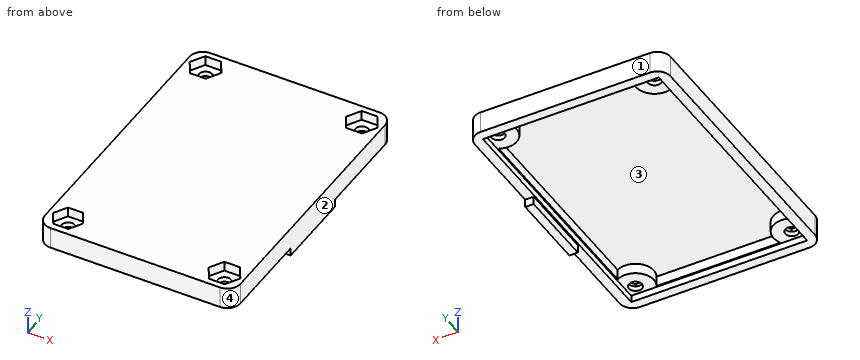
Autodesk Inventor part; units mm, degrees
ref_plane "YZ Plane" through (0, 0, 0) normal (1, 0, 0) x (0, 1, 0)
ref_plane "XZ Plane" through (0, 0, 0) normal (0, 1, 0) x (-1, 0, 0)
ref_plane "XY Plane" through (0, 0, 0) normal (0, 0, 1) x (1, 0, 0)
ref_plane "РабПлоскость1" through (0, 0, 0) normal (0, 0, 1) x (1, 0, 0)
sketch "Эскиз1" plane through (0, 0, 0) normal (0, 0, 1) x (1, 0, 0)
  line L0 (22.5, 29.5) -> (22.5, 9)
  arc A0 (22.5, 29.5) -> (19.5, 32.5) centre (19.5, 29.5) ccw
  line L1 (-19.5, 32.5) -> (19.5, 32.5)
  arc A1 (-19.5, 32.5) -> (-22.5, 29.5) centre (-19.5, 29.5) ccw
  line L2 (-22.5, -29.5) -> (-22.5, 29.5)
  arc A2 (-22.5, -29.5) -> (-19.5, -32.5) centre (-19.5, -29.5) ccw
  line L3 (19.5, -32.5) -> (-19.5, -32.5)
  arc A3 (19.5, -32.5) -> (22.5, -29.5) centre (19.5, -29.5) ccw
  line L4 (22.5, -9) -> (22.5, -29.5)
  line L5 (20, -9) -> (22.5, -9)
  line L6 (20, -25) -> (20, -9)
  line L7 (18, -25) -> (20, -25)
  arc A4 (18, -25) -> (15, -28) centre (18, -28) ccw
  line L8 (15, -30) -> (15, -28)
  line L9 (-15, -30) -> (15, -30)
  line L10 (-15, -28) -> (-15, -30)
  arc A5 (-15, -28) -> (-18, -25) centre (-18, -28) ccw
  line L11 (-20, -25) -> (-18, -25)
  line L12 (-20, 25) -> (-20, -25)
  line L13 (-18, 25) -> (-20, 25)
  arc A6 (-18, 25) -> (-15, 28) centre (-18, 28) ccw
  line L14 (-15, 30) -> (-15, 28)
  line L15 (15, 30) -> (-15, 30)
  line L16 (15, 28) -> (15, 30)
  arc A7 (15, 28) -> (18, 25) centre (18, 28) ccw
  line L17 (20, 25) -> (18, 25)
  line L18 (20, 9) -> (20, 25)
  line L19 (22.5, 9) -> (20, 9)
  circle A8 centre (-18, -28) radius 1.5
  circle A9 centre (-18, 28) radius 1.5
  circle A10 centre (18, 28) radius 1.5
  circle A11 centre (18, -28) radius 1.5
  line L20 (22.5, 9) -> (22.5, -9)
  line L21 (20, 9) -> (20, -9.6142)
  circle A12 centre (18, 28) radius 4.2426
  circle A13 centre (18, -28) radius 4.2426
  circle A14 centre (-18, -28) radius 4.2426
  circle A15 centre (-18, 28) radius 4.2426
  point P0 (0, 0)
  point P1 (-14.2583, -30)
  point P2 (-20, -24.2583)
  point P3 (-20, 24.2583)
  point P4 (-14.2583, 30)
  point P5 (20, -24.2583)
  point P6 (14.2583, -30)
  point P7 (14.2583, 30)
  point P8 (20, 24.2583)
extrude "Выдавливание1" add sketch "Эскиз1" along normal blind 4 contours L0 L19 L18 A12 L15 A15 L12 A14 L9 A13 L6 L5 L4 A3 L3 A2 L2 A1 L1 A0 | L20 L5 L21 L19 | A12 L15 L16 A7 L17 L18 | L18 L17 A7 L16 L15 A12 | A15 L12 L13 A6 L14 L15 | L15 L14 A6 L13 L12 A15 | A13 L9 L8 A4 L7 L6 | L6 L7 A4 L8 L9 A13 | A14 L9 L10 A5 L11 L12 | L12 L11 A5 L10 L9 A14
sketch "Эскиз2" plane through (0, 0, 4) normal (0, 0, 1) x (1, 0, 0)
  circle A0 centre (18, 28) radius 1.5
  circle A1 centre (18, -28) radius 1.5
  circle A2 centre (-18, 28) radius 1.5
  line L0 (16.1813, 24.85) -> (14.3627, 28)
  line L1 (14.3627, 28) -> (16.1813, 31.15)
  line L2 (16.1813, 31.15) -> (19.8187, 31.15)
  line L3 (19.8187, 31.15) -> (21.6373, 28)
  line L4 (21.6373, 28) -> (19.8187, 24.85)
  line L5 (19.8187, 24.85) -> (16.1813, 24.85)
  circle A3 centre (18, -28) radius 1.5
  line L6 (21.6373, -28) -> (19.8187, -31.15)
  line L7 (19.8187, -31.15) -> (16.1813, -31.15)
  line L8 (16.1813, -31.15) -> (14.3627, -28)
  line L9 (14.3627, -28) -> (16.1813, -24.85)
  line L10 (16.1813, -24.85) -> (19.8187, -24.85)
  line L11 (19.8187, -24.85) -> (21.6373, -28)
  line L12 (-14.3627, 28.0054) -> (-16.1766, 24.8527)
  line L13 (-16.1766, 24.8527) -> (-19.8139, 24.8473)
  line L14 (-19.8139, 24.8473) -> (-21.6373, 27.9946)
  line L15 (-21.6373, 27.9946) -> (-19.8234, 31.1473)
  line L16 (-19.8234, 31.1473) -> (-16.1861, 31.1527)
  line L17 (-16.1861, 31.1527) -> (-14.3627, 28.0054)
  line L18 (-16.2701, -24.9933) -> (-14.5312, -27.9948)
  line L19 (-14.5312, -27.9948) -> (-16.2611, -31.0015)
  line L20 (-16.2611, -31.0015) -> (-19.7299, -31.0067)
  line L21 (-19.7299, -31.0067) -> (-21.4688, -28.0052)
  line L22 (-21.4688, -28.0052) -> (-19.7389, -24.9985)
  line L23 (-19.7389, -24.9985) -> (-16.2701, -24.9933)
  line L24 (19.5, 32.5) -> (-19.5, 32.5)
  point P0 (0, 0)
  point P1 (-18, -28)
  point P2 (-18, -28)
  dimension "d2" = 6.3
sketch "Эскиз3" plane through (0, 0, 4) normal (0, 0, 1) x (1, 0, 0)
  line L0 (19.5, 32.5) -> (-19.5, 32.5)
  arc A0 (22.5, 29.5) -> (19.5, 32.5) centre (19.5, 29.5) ccw
  line L1 (22.5, -29.5) -> (22.5, 29.5)
  arc A1 (19.5, -32.5) -> (22.5, -29.5) centre (19.5, -29.5) ccw
  line L2 (-19.5, -32.5) -> (19.5, -32.5)
  arc A2 (-22.5, -29.5) -> (-19.5, -32.5) centre (-19.5, -29.5) ccw
  line L3 (-22.5, 29.5) -> (-22.5, -29.5)
  arc A3 (-19.5, 32.5) -> (-22.5, 29.5) centre (-19.5, 29.5) ccw
  point P0 (0, 0)
extrude "Выдавливание2" add sketch "Эскиз3" along normal blind 1
extrude "Выдавливание3" cut sketch "Эскиз2" along normal blind 1 and the other way blind 1.25 contours A0 | A1 | A2 | L0 L1 L2 L3 L4 L5 | L6 L7 L8 L9 L10 L11 | L12 L13 L14 L15 L16 L17 | L18 L19 L20 L21 L22 L23
sketch "Эскиз4" plane through (0, 0, 0) normal (0, 0, -1) x (-1, 0, 0)
  line L0 (-20.25, -30.25) -> (20.25, -30.25)
  line L1 (20.25, -30.25) -> (20.25, 30.25)
  line L2 (20.25, 30.25) -> (-20.25, 30.25)
  line L3 (-20.25, 30.25) -> (-20.25, -30.25)
  line L4 (-20.25, -30.25) -> (20.25, 30.25) construction
  line L5 (20.25, -30.25) -> (-20.25, 30.25) construction
  point P0 (0, 0)
  dimension "d9" = 40.5
  dimension "d10" = 60.5
extrude "Выдавливание4" cut sketch "Эскиз4" against normal blind 1.6
sketch "Эскиз5" plane through (0, 0, 0) normal (0, 0, -1) x (-1, 0, 0)
  line L0 (-20, 9) -> (-20, -9)
  line L1 (-22.5, 29.5) -> (-22.5, -29.5)
  line L2 (-22.5, -29.5) -> (-22.5, 29.5)
  line L3 (-20, 9) -> (-22.5, 9)
  line L4 (-22.5, 9) -> (-22.5, -9)
  line L5 (-22.5, -9) -> (-20, -9)
  line L6 (-20, -9) -> (-20, 9)
  line L7 (-20.25, -30.25) -> (-20.25, 30.25)
  line L8 (-20.25, -9) -> (-20.55, -9)
  line L9 (-20.55, -9) -> (-20.55, 9)
  point P0 (0, 0)
  dimension "d15" = 0.3
extrude "Выдавливание5" add sketch "Эскиз5" along normal blind 1.85 contours L9 L5 L1 L3
properties part number "bottom"
The listing builds one solid part. Answer for the finished solid, in the listing's coordinates (mm). Face numbers are marked on the shaded views. Coordinates: 2 decimals unless noted, no trailing zeros. Write each loop counter-clockwise with the first axis right and the second up, starting at its lowest first coordinate (ties: lowest second). Pieces come first, ordered by that corner, then holes. Notation, with made-up numbers: (35, -34.5) - (80, -34.5) arc R21 cw to (80, -28.5) - close; hole circle Ø3 at (6.5, 47). An arc over 180 degrees is marked (long way). Put each result on its own line as item: value.
1. The part is cut by section C-C on y = 12. Give the vertices of the cut face in (x, z), plus the area to 3 significant figures.
Answer sheet:
outline: (-22.5, 0) - (-20.25, 0) - (-20.25, 1.6) - (-20, 1.6) - (-20, 4) - (20, 4) - (20, 1.6) - (20.25, 1.6) - (20.25, 0) - (22.5, 0) - (22.5, 5) - (-22.5, 5) - close
area: 64.2 mm^2
2. Determine the mould class of the marked faces 1, 2, 3 and 4 for opening direction Y: pulls with the +Y half, pulls with the -Y half, needs draft (parallel to the pull), parting line crosses it, or undercut.
Answer sheet:
face 1: pulls with the +Y half
face 2: needs draft
face 3: undercut
face 4: pulls with the -Y half
3. The part is cut by section B-B on x = 12. Give the vertices of the cut face in (y, z).
Answer sheet:
outline: (-32.5, 0) - (-30.25, 0) - (-30.25, 1.6) - (-30, 1.6) - (-30, 4) - (30, 4) - (30, 1.6) - (30.25, 1.6) - (30.25, 0) - (32.5, 0) - (32.5, 5) - (-32.5, 5) - close
4. Find the intervals of material crossed by line 1 along X through (y, z) = (28, 2.45); line 2 along Y through (x, z) = (18, 2.4); line 3 along X through (y, z) = (-4, 2), in increasing order. Write a range as from..to.
Answer sheet:
line 1: x = -22.5..-19.5, -16.5..-13.76, 13.76..16.5, 19.5..22.5
line 2: y = -32.5..-29.5, -26.5..-23.76, 23.76..26.5, 29.5..32.5
line 3: x = -22.5..-20, 20..22.5
5. The part is cut by section D-D on y = 5. Give the vertices of the cut face in (x, z), plus the area to 3 significant figures.
Answer sheet:
outline: (-22.5, 0) - (-20.25, 0) - (-20.25, 1.6) - (-20, 1.6) - (-20, 4) - (20, 4) - (20, 1.6) - (20.25, 1.6) - (20.25, 0) - (20.55, 0) - (20.55, -1.85) - (22.5, -1.85) - (22.5, 5) - (-22.5, 5) - close
area: 67.8 mm^2
6. Flat-ended cylindrical pins translate along their axes: pin 1 Ø0.6 at (y, z) = (2.5, -0.5) entering from -X; pin 2 Ø4 at (x, y) = (18, -28) entering from -Z; pin 3 Ø3 at (x, y) = (-0.5, 19) entering from -Z; pin 4 Ø1.8 at (x, y) = (18, 28) entering from +Z. Find the tip coordinate at first contact, or state that the pin passes through.
Answer sheet:
pin 1: stops at x = 20.55
pin 2: stops at z = 1.6
pin 3: stops at z = 4
pin 4: passes through
7. The part is cut by section A-A on x = 18. Give the vertices of the cut face in (y, z), plus the area to 3 significant figures.
Answer sheet:
outline: (-32.5, 0) - (-30.25, 0) - (-30.25, 1.6) - (-29.5, 1.6) - (-29.5, 2.75) - (-31.15, 2.75) - (-31.15, 5) - (-32.5, 5) - close; (-26.5, 1.6) - (-23.76, 1.6) - (-23.76, 4) - (23.76, 4) - (23.76, 1.6) - (26.5, 1.6) - (26.5, 2.75) - (24.85, 2.75) - (24.85, 5) - (-24.85, 5) - (-24.85, 2.75) - (-26.5, 2.75) - close; (29.5, 1.6) - (30.25, 1.6) - (30.25, 0) - (32.5, 0) - (32.5, 5) - (31.15, 5) - (31.15, 2.75) - (29.5, 2.75) - close
area: 78.9 mm^2
